Autodesk Inventor part; units mm, degrees
ref_plane "YZ Plane" through (0, 0, 0) normal (1, 0, 0) x (0, 1, 0)
ref_plane "XZ Plane" through (0, 0, 0) normal (0, 1, 0) x (-1, 0, 0)
ref_plane "XY Plane" through (0, 0, 0) normal (0, 0, 1) x (1, 0, 0)
sketch "Sketch1" plane through (0, 0, 0) normal (0, 0, 1) x (1, 0, 0)
  circle A0 centre (0, 0) radius 101.6
  dimension "d0" = 203.2
extrude "Extrusion1" add sketch "Sketch1" along normal blind 50.8
fillet "Fillet1" radius 19.05 2 edges at (-101.6, 0, 50.8) (-101.6, 0, 0)
sketch "Sketch2" plane through (0, 0, 50.8) normal (0, 0, 1) x (1, 0, 0)
  circle A0 centre (0, 0) radius 82.55
  circle A1 centre (0, 0) radius 25.4
  dimension "d4" = 50.8
extrude "Extrusion2" cut sketch "Sketch2" against normal through all contours A1
properties part number "ShooterWheelConcept"
Verification items for the finished model (mm, model axes). Give positions to 0.01 mm unless a question says otherwise; leave off trailing zeros. Write each loop counter-clockwise with the first axis right and the second up, starting at its lowest first coordinate (ties: lowest second). Pieces come first, ordered by that corner, then holes.
(1) Material ranges on line 1 (Y direction, x = 0, z = 32.5); line 2 (X direction, y = -1, z = 31); line 3 (X direction, y = 17, z = 26), recorded low to high.
(2) Mould release check, pull along Y, two halves, no side actions. Record for faces 1 (the face through (-22.025, 99.184, 25.311)), 2 (the face through (-20, -17, 0)), 3 (the face through (-5.506, -24.796, 25.756)): +Y half, -Y half, draft (parallel to the pull), parting line (faces both ways), or undercut.
(3) Cross-section at D-D (z = 15). Enter the section's corners in (x, y).
(4) Gauge pin test, flat ends, axial feed: pin 1 (3 mm diameter, centred on x = 73.5, y = -56.5, fed in from -Z); pin 2 (2 mm diameter, centred on x = 36, z = 40.5, fed in from -Y); pin 3 (8 mm diameter, centred on x = -45, z = 26.5, fed in from +Y). Record the tip position at first contact, or that the pin passes through.
(5) Cross-section at C-C (z = 39). Enter the section's corners in (x, y), plus the area to 3 significant figures.
(6) Cross-section at A-A (x = 0). Enter the section's corners in (y, z).
Worked out:
1. line 1: y = -101.59 to -25.4, 25.4 to 101.59
1. line 2: x = -101.6 to -25.38, 25.38 to 101.6
1. line 3: x = -100.17 to -18.87, 18.87 to 100.17
2. face 1: parting line
2. face 2: draft
2. face 3: undercut
3. outline: circle Ø202.33 at (0, 0); hole circle Ø50.8 at (0, 0)
4. pin 1: stops at z = 2.08
4. pin 2: stops at y = -93.38
4. pin 3: stops at y = 92.96
5. outline: circle Ø200.33 at (0, 0); hole circle Ø50.8 at (0, 0)
5. area: 29,500 mm2
6. outline: (-101.6, 19.05) arc R19.05 ccw to (-82.55, 0) - (-25.4, 0) - (-25.4, 50.8) - (-82.55, 50.8) arc R19.05 ccw to (-101.6, 31.75) - close; (25.4, 0) - (82.55, 0) arc R19.05 ccw to (101.6, 19.05) - (101.6, 31.75) arc R19.05 ccw to (82.55, 50.8) - (25.4, 50.8) - close
